from build123d import *

# Parameters (mm, degrees)
SKETCH1_W               = 54
SKETCH1_H               = 32
BOSS_EXTRUDE1_DEPTH     = 32
CUT_EXTRUDE1_DEPTH      = 25
CUT_EXTRUDE1_DEPTH_BACK = 25
FILLET1_R               = 1


with BuildPart() as part:
    # Sketch1 → Boss-Extrude1 (new body)
    with BuildSketch(Plane(origin=(0, 0, 0), x_dir=(1, 0, 0), z_dir=(0, 1, 0))):
        Rectangle(SKETCH1_W, SKETCH1_H)
    extrude(amount=BOSS_EXTRUDE1_DEPTH)

    # Sketch2 → Cut-Extrude1 (cut, two sides: drawn at the far end of the back side and taken through both)
    with BuildSketch(Plane(origin=(0, 0, 0), x_dir=(0, 0, -1), z_dir=(1, 0, 0)).offset(-CUT_EXTRUDE1_DEPTH_BACK)):
        with BuildLine():
            Line((-8, 31.5), (-16, 31.5))
            Line((-16, 31.5), (-16, 16.5))
            Line((-16, 16.5), (-8, 16.5))
            ThreePointArc((-8, 16.5), (-0.5, 24), (-8, 31.5))
        make_face()
        with BuildLine():
            Line((16, 16.5), (8, 16.5))
            ThreePointArc((8, 16.5), (0.5, 24), (8, 31.5))
            Line((8, 31.5), (16, 31.5))
            Line((16, 31.5), (16, 16.5))
        make_face()
        with BuildLine():
            Line((16, 0.5), (16, 15.5))
            Line((16, 15.5), (8, 15.5))
            ThreePointArc((8, 15.5), (0.5, 8), (8, 0.5))
            Line((8, 0.5), (16, 0.5))
        make_face()
        with BuildLine():
            Line((-16, 15.5), (-8, 15.5))
            ThreePointArc((-8, 15.5), (-0.5, 8), (-8, 0.5))
            Line((-8, 0.5), (-16, 0.5))
            Line((-16, 0.5), (-16, 15.5))
        make_face()
    extrude(amount=CUT_EXTRUDE1_DEPTH + CUT_EXTRUDE1_DEPTH_BACK, mode=Mode.SUBTRACT)

    # Fillet1
    fillet1_edges = [part.edges().sort_by_distance(p)[0] for p in [
        (27, 32, 0),
        (-25, 24, -16),
        (25, 24, -16),
        (-25, 8, -16),
        (25, 8, -16),
        (-25, 24, 16),
        (25, 24, 16),
        (-27, 32, 0),
        (-25, 8, 16),
        (27, 0, 0),
        (25, 8, 16),
        (-27, 0, 0),
    ]]
    fillet(fillet1_edges, radius=FILLET1_R - 0.0001)  # a hair under: the kernel refuses the full size


solid = part.part
Verification items for the finished model (mm, model axes). A direction names the side the tool comes from. Give positions to 0.01 mm unless a question says otherwise; leave off trailing zeros. Loops run counter-clockwise (first coordinate to the right, second up) from the corner with the lowest first, then second, coordinate; pieces in that order, holes last.
1. Go/stop test with a flat-tipped pin: P1, Ø5, axis at x = 14.5, y = 5, coming from the -Z side. Record where the tip stops, or that it passes through.
Derived:
P1: stops at z = -2.9
2. Release check for a two-part mould opening along X. For faces 1 (the flat face through (0, 31.5, 12)), 2 (the flat face through (-12, 16, 16)), 3 (the flat face through (0, 0.5, -12)), 4 (the flat face through (-27, 16, 0)) record: +X half, -X half, draft (parallel to the pull), parting line (faces both ways), or undercut.
Derived:
face 1: undercut
face 2: draft
face 3: undercut
face 4: -X half
3. Material ranges on probe 1 along Y at (x, z) = (-20, -8.5); probe 2 along X at (y, z) = (24, -12); probe 3 along Y at (x, z) = (-20, 4.5), recorded low to high.
Derived:
probe 1: y = 0 to 0.5, 15.5 to 16.5, 31.5 to 32
probe 2: x = -27 to -25, 25 to 27
probe 3: y = 0 to 1.37, 14.63 to 17.37, 30.63 to 32
4. Cross-section at A-A on y = 3.5. Record the cut outline in (x, z), and give its area (3 significant figures).
Derived:
outline: (-27, -16) - (-26, -16) arc R1 ccw to (-25, -15) - (-25, -2) - (25, -2) - (25, -15) arc R1 ccw to (26, -16) - (27, -16) - (27, 16) - (26, 16) arc R1 ccw to (25, 15) - (25, 2) - (-25, 2) - (-25, 15) arc R1 ccw to (-26, 16) - (-27, 16) - close
area: 327 mm2
5. Tool access check on faces 5 (the flat face through (0, 15.5, 12)), 6 (the cylindrical face through (-0.35, 8.16, -0.5)), 7 (the flat face through (27, 16, 0)). Record the directions out of +Z, -Z, +X, -X, +Y, -Y that give a thin tool (end or side, any length) a straight path to the whole face; none if there is none.
Derived:
face 5: +Z
face 6: -Z
face 7: +Z, -Z, +X, +Y, -Y
6. Cross-section at C-C on x = 16. Record the cut outline in (y, z).
Derived:
outline: (0, -16) - (0.5, -16) - (0.5, -8) arc R7.5 cw to (15.5, -8) - (15.5, -16) - (16.5, -16) - (16.5, -8) arc R7.5 cw to (31.5, -8) - (31.5, -16) - (32, -16) - (32, 16) - (31.5, 16) - (31.5, 8) arc R7.5 cw to (16.5, 8) - (16.5, 16) - (15.5, 16) - (15.5, 8) arc R7.5 cw to (0.5, 8) - (0.5, 16) - (0, 16) - close
7. Cross-section at D-D on y = 24. Record the cut outline in (x, z).
Derived:
outline: (-27, -16) - (-26, -16) arc R1 ccw to (-25, -15) - (-25, -0.5) - (25, -0.5) - (25, -15) arc R1 ccw to (26, -16) - (27, -16) - (27, 16) - (26, 16) arc R1 ccw to (25, 15) - (25, 0.5) - (-25, 0.5) - (-25, 15) arc R1 ccw to (-26, 16) - (-27, 16) - close
8. Cross-section at B-B on z = -3.5. Record the cut outline in (x, y), and give its area (3 significant figures).
Derived:
outline: (-27, 1) arc R1 ccw to (-26, 0) - (26, 0) arc R1 ccw to (27, 1) - (27, 31) arc R1 ccw to (26, 32) - (-26, 32) arc R1 ccw to (-27, 31) - close; hole (-25, 2) - (25, 2) - (25, 14) - (-25, 14) - close; hole (-25, 18) - (25, 18) - (25, 30) - (-25, 30) - close
area: 527 mm2
